For this review, take the finished solid that the model builds, in its own axes (mm). A direction names the side the tool comes from. Round coordinates to 2 decimals unless told otherwise and drop trailing zeros. Order: outer loops, then holes, each group sorted by start corner. A loop starts at its lowest first (then second) coordinate and runs counter-clockwise, first axis right, second up.
```python
from build123d import *

# Parameters (mm, degrees)
SKETCH_281X300_25_R   = 1.6
SKETCH_281X300_25_R_2 = 15
SKETCH_281X300_25_R_3 = 2.15
SKETCH_281X300_25_R_4 = 2.2
F_4MM_DEPTH           = 4
XRU2012_3_4_57_2_R    = 1.7
XRU2012_3_4_57_DEPTH  = 4


with BuildPart() as part:
    # 底板轮廓_281x300_安装孔外移25 → 凸台拉伸_4mm (new body)
    with BuildSketch(Plane.XY):
        with BuildLine():
            Line((-55.5, 108), (-55.5, 142))
            ThreePointArc((-55.5, 142), (-53.156854249, 147.656854249), (-47.5, 150))
            Line((-47.5, 150), (61.5, 150))
            ThreePointArc((61.5, 150), (67.156854249, 147.656854249), (69.5, 142))
            Line((69.5, 142), (69.5, 108))
            ThreePointArc((69.5, 108), (71.843145751, 102.343145751), (77.5, 100))
            Line((77.5, 100), (135.5, 100))
            ThreePointArc((135.5, 100), (139.035533906, 98.535533906), (140.5, 95))
            Line((140.5, 95), (140.5, -95))
            ThreePointArc((140.5, -95), (139.035533906, -98.535533906), (135.5, -100))
            Line((135.5, -100), (77.5, -100))
            ThreePointArc((77.5, -100), (71.843145751, -102.343145751), (69.5, -108))
            Line((69.5, -108), (69.5, -142))
            ThreePointArc((69.5, -142), (67.156854249, -147.656854249), (61.5, -150))
            Line((61.5, -150), (-47.5, -150))
            ThreePointArc((-47.5, -150), (-53.156854249, -147.656854249), (-55.5, -142))
            Line((-55.5, -142), (-55.5, -108))
            ThreePointArc((-55.5, -108), (-57.843145751, -102.343145751), (-63.5, -100))
            Line((-63.5, -100), (-138.5, -100))
            ThreePointArc((-138.5, -100), (-139.914213562, -99.414213562), (-140.5, -98))
            Line((-140.5, -98), (-140.5, -17))
            ThreePointArc((-140.5, -17), (-139.914213562, -15.585786438), (-138.5, -15))
            Line((-138.5, -15), (-132.5, -15))
            ThreePointArc((-132.5, -15), (-131.085786438, -14.414213562), (-130.5, -13))
            Line((-130.5, -13), (-130.5, 97))
            ThreePointArc((-130.5, 97), (-129.621320344, 99.121320344), (-127.5, 100))
            Line((-127.5, 100), (-63.5, 100))
            ThreePointArc((-63.5, 100), (-57.843145751, 102.343145751), (-55.5, 108))
        make_face()
        with Locations((100.5, -61)):
            Circle(SKETCH_281X300_25_R, mode=Mode.SUBTRACT)
        with Locations((130.5, -61)):
            Circle(SKETCH_281X300_25_R, mode=Mode.SUBTRACT)
        with Locations((100.5, 61)):
            Circle(SKETCH_281X300_25_R, mode=Mode.SUBTRACT)
        with Locations((7, 90.5)):
            Circle(SKETCH_281X300_25_R_2, mode=Mode.SUBTRACT)
        with Locations((7, 140)):
            Circle(SKETCH_281X300_25_R_3, mode=Mode.SUBTRACT)
        with Locations((-42.5, 90.5)):
            Circle(SKETCH_281X300_25_R_3, mode=Mode.SUBTRACT)
        with Locations((56.5, 90.5)):
            Circle(SKETCH_281X300_25_R_3, mode=Mode.SUBTRACT)
        with Locations((-40, 140)):
            Circle(SKETCH_281X300_25_R_3, mode=Mode.SUBTRACT)
        with Locations((130.5, 61)):
            Circle(SKETCH_281X300_25_R, mode=Mode.SUBTRACT)
        with Locations((49, 140)):
            Circle(SKETCH_281X300_25_R_3, mode=Mode.SUBTRACT)
        with Locations((7, 41)):
            Circle(SKETCH_281X300_25_R_3, mode=Mode.SUBTRACT)
        with Locations((31.290367902, -137.395183951)):
            Circle(SKETCH_281X300_25_R_4, mode=Mode.SUBTRACT)
        with Locations((-17.5, -137.395183951)):
            Circle(SKETCH_281X300_25_R_4, mode=Mode.SUBTRACT)
        with Locations((-17.5, -88.604816049)):
            Circle(SKETCH_281X300_25_R_4, mode=Mode.SUBTRACT)
        with Locations((31.290367902, -88.604816049)):
            Circle(SKETCH_281X300_25_R_4, mode=Mode.SUBTRACT)
        with Locations((7, 111.5)):
            Circle(SKETCH_281X300_25_R, mode=Mode.SUBTRACT)
        with Locations((25.186533479, 101)):
            Circle(SKETCH_281X300_25_R, mode=Mode.SUBTRACT)
        with Locations((100.5, -91)):
            Circle(SKETCH_281X300_25_R, mode=Mode.SUBTRACT)
        with Locations((25.186533479, 80)):
            Circle(SKETCH_281X300_25_R, mode=Mode.SUBTRACT)
        with Locations((100.5, 91)):
            Circle(SKETCH_281X300_25_R, mode=Mode.SUBTRACT)
        with Locations((7, 69.5)):
            Circle(SKETCH_281X300_25_R, mode=Mode.SUBTRACT)
        with Locations((130.5, 91)):
            Circle(SKETCH_281X300_25_R, mode=Mode.SUBTRACT)
        with Locations((130.5, -91)):
            Circle(SKETCH_281X300_25_R, mode=Mode.SUBTRACT)
        with Locations((-43, -105)):
            Circle(SKETCH_281X300_25_R, mode=Mode.SUBTRACT)
        with Locations((57, -57)):
            Circle(SKETCH_281X300_25_R, mode=Mode.SUBTRACT)
        with Locations((-43, -57)):
            Circle(SKETCH_281X300_25_R, mode=Mode.SUBTRACT)
        with Locations((57, -105)):
            Circle(SKETCH_281X300_25_R, mode=Mode.SUBTRACT)
        with Locations((-11.186533479, 80)):
            Circle(SKETCH_281X300_25_R, mode=Mode.SUBTRACT)
        with Locations((-11.186533479, 101)):
            Circle(SKETCH_281X300_25_R, mode=Mode.SUBTRACT)
        with Locations((130.5, 10)):
            Circle(SKETCH_281X300_25_R, mode=Mode.SUBTRACT)
        with Locations((130.5, -10)):
            Circle(SKETCH_281X300_25_R, mode=Mode.SUBTRACT)
        with Locations((-120.5, 10)):
            Circle(SKETCH_281X300_25_R, mode=Mode.SUBTRACT)
        with Locations((-120.5, -10)):
            Circle(SKETCH_281X300_25_R, mode=Mode.SUBTRACT)
        with Locations((-43, -115)):
            Circle(SKETCH_281X300_25_R, mode=Mode.SUBTRACT)
        with Locations((57, -67)):
            Circle(SKETCH_281X300_25_R, mode=Mode.SUBTRACT)
        with Locations((57, -115)):
            Circle(SKETCH_281X300_25_R, mode=Mode.SUBTRACT)
        with Locations((-43, -67)):
            Circle(SKETCH_281X300_25_R, mode=Mode.SUBTRACT)
        with Locations((-120.5, -91)):
            Circle(SKETCH_281X300_25_R, mode=Mode.SUBTRACT)
        with Locations((-90.5, -91)):
            Circle(SKETCH_281X300_25_R, mode=Mode.SUBTRACT)
        with Locations((-120.5, 91)):
            Circle(SKETCH_281X300_25_R, mode=Mode.SUBTRACT)
        with Locations((-90.5, 91)):
            Circle(SKETCH_281X300_25_R, mode=Mode.SUBTRACT)
        with Locations((-90.5, 61)):
            Circle(SKETCH_281X300_25_R, mode=Mode.SUBTRACT)
        with Locations((-120.5, 61)):
            Circle(SKETCH_281X300_25_R, mode=Mode.SUBTRACT)
        with Locations((-90.5, -61)):
            Circle(SKETCH_281X300_25_R, mode=Mode.SUBTRACT)
        with Locations((-120.5, -61)):
            Circle(SKETCH_281X300_25_R, mode=Mode.SUBTRACT)
        with BuildLine():
            Line((-25.5, -97), (-25.5, -129))
            ThreePointArc((-25.5, -129), (-24.914213562, -130.414213562), (-23.5, -131))
            Line((-23.5, -131), (42.5, -131))
            ThreePointArc((42.5, -131), (43.914213562, -130.414213562), (44.5, -129))
            Line((44.5, -129), (44.5, -97))
            ThreePointArc((44.5, -97), (43.914213562, -95.585786438), (42.5, -95))
            Line((42.5, -95), (-23.5, -95))
            ThreePointArc((-23.5, -95), (-24.914213562, -95.585786438), (-25.5, -97))
        make_face(mode=Mode.SUBTRACT)
        with BuildLine():
            Line((75.5, 50), (75.5, 36))
            ThreePointArc((75.5, 36), (80.5, 31), (85.5, 36))
            Line((85.5, 36), (85.5, 50))
            ThreePointArc((85.5, 50), (80.5, 55), (75.5, 50))
        make_face(mode=Mode.SUBTRACT)
        with BuildLine():
            Line((85.5, -50), (85.5, -36))
            ThreePointArc((85.5, -36), (80.5, -31), (75.5, -36))
            Line((75.5, -36), (75.5, -50))
            ThreePointArc((75.5, -50), (80.5, -55), (85.5, -50))
        make_face(mode=Mode.SUBTRACT)
        with BuildLine():
            Line((-95.5, -10), (-75.5, -10))
            ThreePointArc((-75.5, -10), (-65.5, 0), (-75.5, 10))
            Line((-75.5, 10), (-95.5, 10))
            ThreePointArc((-95.5, 10), (-105.5, 0), (-95.5, -10))
        make_face(mode=Mode.SUBTRACT)
    extrude(amount=F_4MM_DEPTH)

    # XRU2012__3.4___57 2 → XRU2012__3.4___57 (cut)
    with BuildSketch(Plane.XY.offset(4)):
        with Locations((35.5, 90.5)):
            Circle(XRU2012_3_4_57_2_R)
        with Locations((21.25, 115.181724008)):
            Circle(XRU2012_3_4_57_2_R)
        with Locations((-7.25, 115.181724008)):
            Circle(XRU2012_3_4_57_2_R)
        with Locations((-21.5, 90.5)):
            Circle(XRU2012_3_4_57_2_R)
        with Locations((-7.25, 65.818275992)):
            Circle(XRU2012_3_4_57_2_R)
        with Locations((21.25, 65.818275992)):
            Circle(XRU2012_3_4_57_2_R)
    extrude(amount=-XRU2012_3_4_57_DEPTH, mode=Mode.SUBTRACT)


solid = part.part
```
Q1. Take a section at C-C, the plane x = 82. State the section outline as (y, z) points, plus the area to 3 significant figures.
Q2. Take a section at A-A, the plane x = -83.5. State the section outline as (y, z) points, plus the area to 3 significant figures.
Q3. Clearance check with flat-ended pins moving along their axes: pin 1 (1.5 mm diameter, centred on x = -61, z = 1.5, fed in from +Y); pin 2 (3 mm diameter, centred on x = 25.19, y = 80, fed in from -Z). State where each tip first meets the part, or that it passes through.
Q4. Take a section at D-D, the plane z = 2.6. Count the separate pieces of the cut face and the enclosed holes in it, plus the area to 3 significant figures.
Q5. Take a section at B-B, the plane y = 1. State the section outline as (x, z) points.
Q6. Wall thickness on line 1 (X direction, y = -115, z = 2.9); line 2 (Y direction, x = 100.5, z = 1.05); line 3 (Y direction, x = -43, z = 2.6): over which ranges is each line inside the solid? List them lowest first.
Q7. Tool access review of faces 4 (the face through (2, 2, 4)), 5 (the face through (-65.5, -0.2, 2)): name each direction out of +Z, -Z, +X, -X, +Y, -Y from which nothing blocks a thin tool from reaching the whole face with its end or side.
Q8. Mouldability with a two-part tool opening along Y and no side actions: class faces 1 (the face through (-53.094, -147.719, 1.972)), 2 (the face through (-57.906, 102.281, 1.972)), 3 (the face through (3.748, 75.857, 1.972)) as +Y half, -Y half, draft (parallel to the pull), parting line (faces both ways), or undercut.
Working result:
1. outline: (-100, 0) - (-54.77, 0) - (-54.77, 4) - (-100, 4) - close; (-31.23, 0) - (31.23, 0) - (31.23, 4) - (-31.23, 4) - close; (54.77, 0) - (100, 0) - (100, 4) - (54.77, 4) - close
1. area: 612 mm2
2. outline: (-100, 0) - (-10, 0) - (-10, 4) - (-100, 4) - close; (10, 0) - (100, 0) - (100, 4) - (10, 4) - close
2. area: 720 mm2
3. pin 1: stops at y = 100.69
3. pin 2: passes through
4. separate pieces: 1
4. enclosed holes: 55
4. area: 62,700 mm2
5. outline: (-130.5, 0) - (-105.45, 0) - (-105.45, 4) - (-130.5, 4) - close; (-65.55, 0) - (140.5, 0) - (140.5, 4) - (-65.55, 4) - close
6. line 1: x = -55.5 to -44.6, -41.4 to -25.5, 44.5 to 55.4, 58.6 to 69.5
6. line 2: y = -100 to -92.6, -89.4 to -62.6, -59.4 to 59.4, 62.6 to 89.4, 92.6 to 100
6. line 3: y = -150 to -116.6, -113.4 to -106.6, -103.4 to -68.6, -65.4 to -58.6, -55.4 to 88.41, 92.59 to 150
7. face 4: +Z, +X, -X, +Y, -Y
7. face 5: +Z, -Z
8. face 1: -Y half
8. face 2: +Y half
8. face 3: undercut
